Could you check a few things on this model? Use its own coordinates, in mm. Face numbers are marked on the shaded views. A direction names the side the tool comes from. Round coordinates to 2 decimals unless told otherwise and drop trailing zeros. Loops run counter-clockwise (first coordinate to the right, second up) from the corner with the lowest first, then second, coordinate; pieces in that order, holes last. Notation, with made-up numbers: (9.25, 57.25) - (50.25, 57.25) arc R29 ccw to (50.25, 77.25) - close; hole circle Ø1 at (-12, 28). An arc over 180 degrees is marked (long way). Answer as CSV lines item,"result". Start each with the question number.
1) Suppose I cut it at A-A, the plane z = -7.5. Write out the boundary of the cut face in (x, y).
2) Which directions (+Z, -Z, +X, -X, +Y, -Y) give clear straight access to the entire face, cutting with the end or side of a thin tool? Please do the marked faces 1, 2 and 3.
3) Please list where these lines run through material, in increasing order: line 1 along X through (y, z) = (1, 0.75); line 2 along Y through (x, z) = (-2, 2.25); line 3 along Z through (x, y) = (-2.75, -1).
4) I'm going to push a flat-ended pin straight in: pin 1 Ø2 at (x, z) = (2.5, -3.5) entering from -Y. Where does the tip first touch, or does it pass through?
5) We'd pull the mould along Y, two halves only. Please class the marked faces 4, 5 and 6: pulls with the +Y half, pulls with the -Y half, needs draft (parallel to the pull), parting line crosses it, or undercut.
Autodesk Fusion 360 part; units mm, degrees
sketch "Sketch1" plane through (0, 0, 0) normal (0, 1, 0) x (1, 0, 0)
  line L0 (-2.1, 0) -> (-2.1, 13)
  line L1 (-2.1, 13) -> (0, 13)
  line L2 (0, 13) -> (0, -3.1)
  line L3 (-2.1, 0) -> (-4, 0)
  line L4 (-4, 0) -> (-4, -1.7235)
  arc A0 (-4, -1.7235) -> (0, -3.1) centre (0, 3.4) ccw
  dimension "d9" = 4.2
  dimension "d74" = 13
  dimension "d75" = 8
  dimension "d78" = 3.1
  dimension "d118" = 6.5
revolve "Revolve1" add sketch "Sketch1" angle 360 about axis through (0, 0, -13) along (0, 0, 1) makes body 1
ref_plane "WorkPlane1" through (0, 0, 3.1) normal (0, 0, 1) x (1, 0, 0)
sketch "Sketch7" plane through (0, 0, 3.1) normal (0, 0, 1) x (1, 0, 0)
  line L0 (-0.618, 0.618) -> (0.618, 0.618)
  line L1 (0.618, 0.618) -> (0.618, -0.618)
  line L2 (0.618, -0.618) -> (-0.618, -0.618)
  line L3 (-0.618, -0.618) -> (-0.618, 0.618)
  point P0 (-0.618, 0)
  point P1 (0, 0.618)
  dimension "d65" = 1.236
  dimension "d119" = 1.236
extrude "Extrude4" add sketch "Sketch7" against normal blind 2.032 draft -10 separate body makes body 2
sketch "Sketch10" plane through (0, 0, 3.1) normal (0, 0, 1) x (1, 0, 0)
  line L0 (-2.18, 0) -> (2.18, 0) construction
  line L1 (-2.18, 0.515) -> (2.18, 0.515)
  line L2 (2.18, 0.515) -> (2.18, -0.515)
  line L3 (2.18, -0.515) -> (-2.18, -0.515)
  line L4 (-2.18, -0.515) -> (-2.18, 0.515)
  line L5 (0.515, -2.18) -> (-0.515, -2.18)
  line L6 (-0.515, -2.18) -> (-0.515, 2.18)
  line L7 (0.515, 2.18) -> (0.515, -2.18)
  line L8 (-0.515, 2.18) -> (0.515, 2.18)
  dimension "d90" = 4.36
  dimension "d91" = 1.03
  dimension "d114" = 90
extrude "Extrude1" add sketch "Sketch10" against normal blind 2.54 draft -6 separate body makes body 3 at (-0.426, -1.536, 2.2533)
draft "Draft2" angle 30 neutral plane through (0, 0, 3.1) pull (0, 0, 1) 4 faces at (0.0827, 2.091, 2.2533) (2.091, -0.0827, 2.2533) (-2.091, 0.0827, 2.2533) (-0.0827, -2.091, 2.2533) on bodies 3
combine "Combine1" operation cut target body 1 tool bodies 2 3
ref_plane "WorkPlane2" through (-0.4816, 1.9491, 2.7822) normal (0, 0, -1) x (-1, 0, 0)
sketch "Sketch8" plane through (-0.2873, 1.3933, 2.7822) normal (0, 0, -1) x (1, 0, 0)
  line L0 (0.2873, 1.3933) -> (1.983, 3.089)
  line L1 (2.0373, 1.3933) -> (22.7873, 1.3933)
  point P0 (0.2873, 1.3933)
  dimension "d83" = 2.398
  dimension "d112" = 45
ref_plane "WorkPlane3" through (0.8478, -0.8478, 2.7822) normal (-0.6645, -0.6645, 0.342) x (0.7071, -0.7071, 0)
sketch "Sketch9" plane through (0.4897, -0.7159, 2.3426) normal (-0.6645, -0.6645, 0.342) x (0.7071, -0.7071, 0)
  line L0 (-0.8525, 0.4678) -> (1.5455, 0.4678)
  line L1 (1.5455, 0.4678) -> (1.5455, 2.5278)
  line L2 (1.5455, 2.5278) -> (-0.8525, 2.5278)
  line L3 (-0.8525, 2.5278) -> (-0.8525, 0.4678)
  point P0 (-0.8525, 0.4678)
  point P1 (1.5455, 0.4678)
  dimension "d85" = 2.06
extrude "Extrude6" cut sketch "Sketch9" along normal blind 0.515 draft -50 bodies 1
pattern_circular "C-Pattern1" count 4 over 360 about axis through (0, 0, 1.75) along (0, 0, 1) of "Extrude6"
fillet "Fillet4" radius 1.0333 1 edges at (-3.7293, 1.4465, 1.7235) on bodies 1
thread "Thread2" thread offset 0 thread length 11.6
sketch "Sketch5" plane through (0, 0, 0) normal (0, 1, 0) x (1, 0, 0)
  line L0 (0, 13) -> (0, -3.1)
  line L1 (0, 13) -> (-2.142, 13)
  line L2 (-2.142, 13) -> (-2.142, 7.9301)
  line L3 (-2.142, 7.9301) -> (0, 13)
  dimension "d109" = 5.0699
  dimension "d111" = 2.142
revolve "Revolve2" cut sketch "Sketch5" angle 360 about axis through (0, 0, 1.75) along (0, 0, 1) bodies 1
equation "d9 = adsk_nomdia"
equation "adsk_nomlen = 13.00 mm"
equation "adsk_headh = 3.10 mm"
equation "adsk_headdia = 8.00 mm"
equation "adsk_nomdia = 4.20 mm"
equation "adsk_phildia = 4.36 mm"
equation "adsk_philwidth = 1.03 mm"
equation "adsk_phildepth = 2.54 mm"
equation "d65 = adsk_philwidth * 1.2"
equation "d68 = -adsk_phildepth * 0.8"
equation "d74 = adsk_nomlen"
equation "d75 = adsk_headdia"
equation "d78 = adsk_headh"
equation "d79 = adsk_headh"
equation "d83 = adsk_phildia / 2 * 1.1"
equation "d85 = adsk_philwidth * 2"
equation "d86 = adsk_philwidth / 2"
equation "d90 = adsk_phildia"
equation "d91 = adsk_philwidth"
equation "adsk_startlen = 5.069855 mm"
equation "adsk_thrlen = 11.60 mm"
equation "d102 = adsk_headh / 3"
equation "d104 = adsk_thrlen"
equation "d109 = adsk_startlen"
equation "d111 = adsk_nomdia * 0.51"
equation "adsk_ovalrad = 6.50 mm"
equation "d118 = adsk_ovalrad"
equation "d119 = adsk_philwidth * 1.2"
properties part number "CRPHTS ANSI B18.6.5M - 4.2 x 1.4 x 13  - AB - IA Steel Grade 2 Plain"
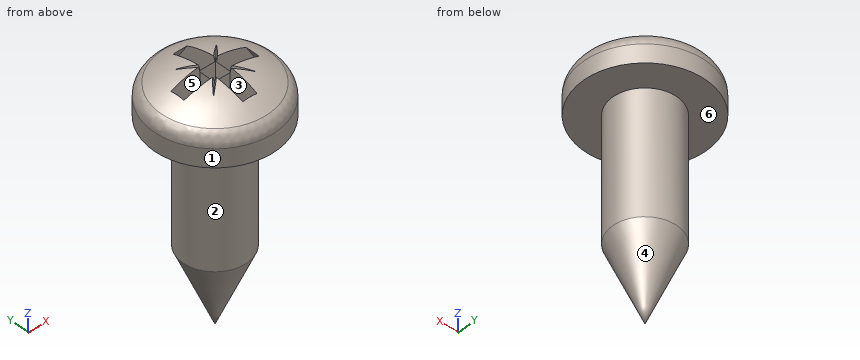
Filled sheet:
1,outline,"circle Ø4.2 at (0, 0)"
2,face 1,"+Z, -Z"
2,face 2,"-Z"
2,face 3,"none"
3,line 1,"-3.87 to -0.27, 0.27 to 3.87"
3,line 2,"-2.52 to -0.43, 0.43 to 2.52"
3,line 3,"0 to 2.4"
4,pin 1,"y = -1.47"
5,face 4,"parting line crosses it"
5,face 5,"undercut"
5,face 6,"needs draft"
